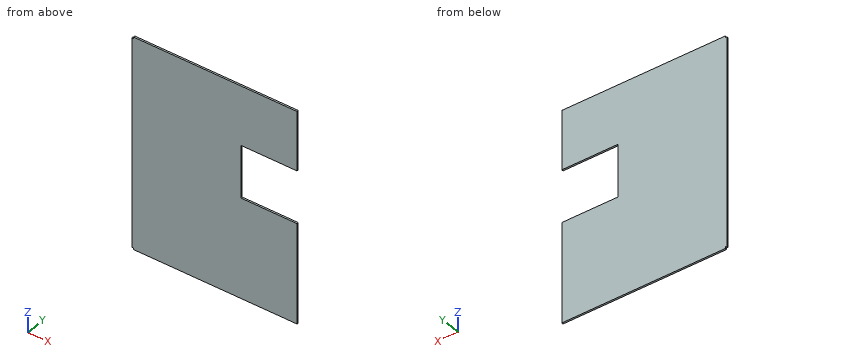
Autodesk Inventor part; units mm, degrees
ref_plane "YZ Plane" through (0, 0, 0) normal (1, 0, 0) x (0, 1, 0)
ref_plane "XZ Plane" through (0, 0, 0) normal (0, 1, 0) x (-1, 0, 0)
ref_plane "XY Plane" through (0, 0, 0) normal (0, 0, 1) x (1, 0, 0)
sketch "Эскиз1" plane through (0, 0, 0) normal (0, 1, 0) x (-1, 0, 0)
  line L0 (0, 0) -> (388, 0)
  line L1 (388, 0) -> (388, -508)
  line L2 (388, -508) -> (0, -508)
  line L3 (0, -508) -> (0, 0)
  dimension "d0" = 388
  dimension "d1" = 508
extrude "Выдавливание1" add sketch "Эскиз1" along normal blind 4
sketch "Эскиз2" plane through (0, 4, 0) normal (0, 1, 0) x (1, 0, 0)
  line L0 (0, 0) -> (0, 508)
  line L1 (0, 142) -> (-132, 142)
  line L2 (-132, 142) -> (-132, 268)
  line L3 (-132, 268) -> (0, 268)
  line L4 (0, 268) -> (0, 142)
  line L5 (-388, 0) -> (0, 0)
  point P0 (0, 268)
  dimension "d4" = 132
  dimension "d5" = 126
  dimension "d6" = 142
extrude "Выдавливание2" cut sketch "Эскиз2" against normal blind 4
sketch "Эскиз3" plane through (0, 4, 0) normal (0, 1, 0) x (1, 0, 0)
  line L0 (-388, 0) -> (0, 0)
  line L1 (-388, 0) -> (-384, 0)
  line L2 (-384, 0) -> (-384, 4)
  line L3 (-384, 4) -> (-388, 4)
  line L4 (-388, 4) -> (-388, 0)
  line L5 (-388, 508) -> (-388, 0)
  line L6 (-388, 508) -> (-384, 508)
  line L7 (-384, 508) -> (-384, 504)
  line L8 (-384, 504) -> (-388, 504)
  line L9 (-388, 504) -> (-388, 508)
  dimension "d9" = 4
  dimension "d10" = 4
  dimension "d11" = 4
  dimension "d12" = 4
extrude "Выдавливание3" cut sketch "Эскиз3" against normal blind 4
properties part number "MountingWallSide"
Could you check a few things on this model? Use its own coordinates, in mm. Round coordinates to 2 decimals unless told otherwise and drop trailing zeros. Loops run counter-clockwise (first coordinate to the right, second up) from the corner with the lowest first, then second, coordinate; pieces in that order, holes last. Notation, with made-up numbers: M 57,14 L 70,14 A16 ccw 70,40 Z; hole C 29.25,-3.75 d10. An arc over 180 degrees is marked long. Put each result on its own line as item: value.
Q1. For pin 1 (2 mm diameter, centred on x = -385.5, y = 1, fed in from +Z); pin 2 (1.2 mm diameter, centred on y = 2.5, z = -220.5, fed in from +X); pin 3 (2 mm diameter, centred on x = -387, y = 2, fed in from -Z), each with a flat end and sliding along its axis, tell me the tip position at first contact or that it passes through.
Check result:
pin 1: z = -4
pin 2: x = -132
pin 3: z = -504
Q2. Imagine slicing it at B-B (y = 2). Write out the boundary of the cut face in (x, z).
Check result:
outline: M -388,-504 L -384,-504 L -384,-508 L 0,-508 L 0,-268 L -132,-268 L -132,-142 L 0,-142 L 0,0 L -384,0 L -384,-4 L -388,-4 Z
Q3. Imagine slicing it at A-A (x = -61.5). Write out the boundary of the cut face in (y, z), then the cut area to 3 significant figures.
Check result:
outline: M 0,-508 L 4,-508 L 4,-268 L 0,-268 Z; M 0,-142 L 4,-142 L 4,0 L 0,0 Z
area: 1,530 mm2
Q4. I need wall thicknesses on probe 1 along Z at (x, y) = (-60.5, 0.4); probe 2 along X at (y, z) = (1.6, -184). Which ranges of each line are inside material? Lowest first, please.
Check result:
probe 1: -508 to -268, -142 to 0
probe 2: -388 to -132
Q5. Imagine slicing it at C-C (z = -206.5). Write out the boundary of the cut face in (x, y), then the cut area to 3 significant figures.
Check result:
outline: M -388,0 L -132,0 L -132,4 L -388,4 Z
area: 1,020 mm2
